```python
from build123d import *

# Parameters (mm, degrees)
F1_DEPTH = 3


with BuildPart() as f1:
    # F0 (on Top) → F1 (new body)
    with BuildSketch(Plane.XY):
        Polygon((-36.8060796608, 21.25), (0, 85), (-11, 85), (-4.0717967697, 81), (-12.0717967697, 67.1435935394), (-19, 71.1435935394), (-45.0560796608, 26.0131397208), align=None)
        Polygon((0, 0), (0, 85), (-36.8060796608, 21.25), align=None)
        Polygon((36.8060796608, 21.25), (0, 85), (0, 0), align=None)
        Polygon((11, 85), (0, 85), (36.8060796608, 21.25), (45.0560796608, 26.0131397208), (19, 71.1435935394), (12.0717967697, 67.1435935394), (4.0717967697, 81), align=None)
        Polygon((45.0560796608, 26.0131397208), (36.8060796608, 21.25), (73.6121593217, -42.5), (79.1121593217, -32.9737205584), (72.1839560914, -36.9737205584), (64.1839560914, -23.1173140978), (71.1121593217, -19.1173140978), align=None)
        Polygon((73.6121593217, -42.5), (36.8060796608, 21.25), (0, 0), align=None)
        Polygon((73.6121593217, -42.5), (0, 0), (-73.6121593217, -42.5), align=None)
        Polygon((0, 0), (-36.8060796608, 21.25), (-73.6121593217, -42.5), align=None)
        Polygon((-73.6121593217, -42.5), (-36.8060796608, 21.25), (-45.0560796608, 26.0131397208), (-71.1121593217, -19.1173140978), (-64.1839560914, -23.1173140978), (-72.1839560914, -36.9737205584), (-79.1121593217, -32.9737205584), align=None)
        Polygon((68.1121593217, -52.0262794416), (73.6121593217, -42.5), (-73.6121593217, -42.5), (-68.1121593217, -52.0262794416), (-68.1121593217, -44.0262794416), (-52.1121593217, -44.0262794416), (-52.1121593217, -52.0262794416), (52.1121593217, -52.0262794416), (52.1121593217, -44.0262794416), (68.1121593217, -44.0262794416), align=None)
    extrude(amount=F1_DEPTH)


solid = f1.part
```
Design review of the part built by this model. Coordinates are the model's own, in mm. A direction names the side the tool comes from. Round coordinates to 2 decimals unless told otherwise and drop trailing zeros. Write each loop counter-clockwise with the first axis right and the second up, starting at its lowest first coordinate (ties: lowest second). Pieces come first, ordered by that corner, then holes. Notation, with made-up numbers: (-11, -39.5) -> (-4, -39.5) arc R19 cw to (-4, -22.5) -> close; hole circle Ø4 at (-6.75, -18). An arc over 180 degrees is marked (long way). Answer in a Markdown table with one row per item.
Q1. To check wall thickness, follow L1, parallel to X at y = -35, z = 2.1; L2, parallel to X at y = -35.5, z = 0.6; L3, parallel to Y at x = 9, z = 1.45. State the ranges of each line that lie inside material, in increasing order. Write a range as [from, to].
The answers:
| item | result |
|---|---|
| L1 | [-77.94, -75.6], [-71.04, 71.04], [75.6, 77.94] |
| L2 | [-77.65, -74.74], [-71.33, 71.33], [74.74, 77.65] |
| L3 | [-52.03, 72.46], [83.85, 85] |
Q2. Take a section at C-C, the plane x = -57. State the section outline as (y, z) points.
The answers:
| item | result |
|---|---|
| outline | (-44.03, 0) -> (5.33, 0) -> (5.33, 3) -> (-44.03, 3) -> close |
Q3. Take a section at A-A, the plane z = 2. State the section outline as (x, y) points, then the cut area to 3 significant figures.
The answers:
| item | result |
|---|---|
| outline | (-79.11, -32.97) -> (-68.11, -52.03) -> (-68.11, -44.03) -> (-52.11, -44.03) -> (-52.11, -52.03) -> (52.11, -52.03) -> (52.11, -44.03) -> (68.11, -44.03) -> (68.11, -52.03) -> (79.11, -32.97) -> (72.18, -36.97) -> (64.18, -23.12) -> (71.11, -19.12) -> (19, 71.14) -> (12.07, 67.14) -> (4.07, 81) -> (11, 85) -> (-11, 85) -> (-4.07, 81) -> (-12.07, 67.14) -> (-19, 71.14) -> (-71.11, -19.12) -> (-64.18, -23.12) -> (-72.18, -36.97) -> close |
| area | 12,700 mm² |
Q4. For faces 5 (the face through (8.13, 73.97, 1.48)), 6 (the face through (-7.584, 83.028, 1.479)), 7 (the face through (7.487, 82.972, 1.479)), 8 (the face through (-15.487, 69.116, 1.479)), list the 3-axis set-ups (+Z, -Z, +X, -X, +Y, -Y) from which the entire face can be reached by the end or side of a thin tool; tool diameter is ignored.
The answers:
| item | result |
|---|---|
| face 5 | +Z, -Z |
| face 6 | +Z, -Z, -X |
| face 7 | +Z, -Z, +X |
| face 8 | +Z, -Z, +Y |
Q5. Take a section at B-B, the plane y = -29. State the section outline as (x, z) points, then the cut area to 3 significant figures.
The answers:
| item | result |
|---|---|
| outline | (-67.58, 0) -> (67.58, 0) -> (67.58, 3) -> (-67.58, 3) -> close |
| area | 405 mm² |
Q6. Clearance check with flat-ended pins moving along their axes: pin 1 Ø1.5 at (y, z) = (-31.5, 1.5) entering from +X; pin 2 Ø1.5 at (y, z) = (-49.5, 1.5) entering from -X; pin 3 Ø1 at (y, z) = (3.5, 1.5) entering from +X; pin 4 Ø12 at (x, y) = (-36, 57.5) entering from +Z. State where each tip first meets the part, or that it passes through.
The answers:
| item | result |
|---|---|
| pin 1 | x = 69.46 |
| pin 2 | x = -70 |
| pin 3 | x = 58.34 |
| pin 4 | through |
Q7. Draft analysis for pull direction Y (two halves, no side actions). For faces 1 (the face through (-75.6, -35, 1.5)), 2 (the face through (-1, 2, 3)), 3 (the face through (-8, 74.2, 1.5)), 4 (the face through (73.535, -42.633, 1.479)), state which applies: +Y half, -Y half, draft (parallel to the pull), parting line (faces both ways), or undercut.
The answers:
| item | result |
|---|---|
| face 1 | +Y half |
| face 2 | draft |
| face 3 | undercut |
| face 4 | -Y half |
